The listing builds one solid part. Answer for the finished solid, in the listing's coordinates (mm). A direction names the side the tool comes from. Coordinates: 2 decimals unless noted, no trailing zeros. Order: outer loops, then holes, each group sorted by start corner. A loop starts at its lowest first (then second) coordinate and runs counter-clockwise, first axis right, second up. Notation, with made-up numbers: (25.5, -8.75) -> (45.5, -8.75) arc R13 cw to (45.5, 8.25) -> close; hole circle Ø3 at (54.5, -7). An arc over 180 degrees is marked (long way). Put each result on its own line as item: value. Start each with the question number.
```python
from build123d import *

# Parameters (mm, degrees)
BOSS_EXTRUDE1_DEPTH = 3.175
SKETCH2_R           = 1.6
CUT_EXTRUDE1_DEPTH  = 3.175


with BuildPart() as part:
    # Sketch1 → Boss-Extrude1 (new body)
    with BuildSketch(Plane.XY):
        Polygon((25, 7.5), (-25, 7.5), (-25, -7.5), (-17.5, -7.5), (-17.5, -10.675), (-12.5, -10.675), (-12.5, -7.5), (-2.5, -7.5), (-2.5, -10.675), (2.5, -10.675), (2.5, -7.5), (12.5, -7.5), (12.5, -10.675), (17.5, -10.675), (17.5, -7.5), (25, -7.5), align=None)
    extrude(amount=BOSS_EXTRUDE1_DEPTH)

    # Sketch2 → Cut-Extrude1 (cut)
    with BuildSketch(Plane.XY.offset(3.175)):
        with Locations((-18.4, 0)):
            Circle(SKETCH2_R)
        with Locations((18.4, 0)):
            Circle(SKETCH2_R)
    extrude(amount=-CUT_EXTRUDE1_DEPTH, mode=Mode.SUBTRACT)


solid = part.part
```
(1) Find the intervals of material crossed by L1, parallel to X at y = -9.25, z = 1.7; L2, parallel to Y at x = -18.4, z = 1.7; L3, parallel to X at y = 0.5, z = 2.95, in increasing order.
(2) The part is cut by section B-B on y = -9. Determine the outline of the cut face in (x, z) (3 decimals).
(3) Each of these flat-tipped pins is pushed along its axis until it touches: P1, Ø1, axis at y = -9.5, z = 2, coming from the +X side; P2, Ø1, axis at y = -9, z = 1.5, coming from the -X side; P3, Ø1, axis at x = 20, z = 2, coming from the -Y side. Where does it stop, or does it pass through?
(4) A tool of negligible diameter and unlimited length cuts with its end or side. For faces 1 (the flat face through (7, -7.5, 2)), 2 (the flat face through (-21, -7.5, 2)), 3 (the flat face through (0, 1, 0)), 4 (the flat face through (21, -7.5, 2)), from which of +Z, -Z, +X, -X, +Y, -Y can it reach the whole face along a straight path? Write none if from no direction.
(5) For a pull along X with two mould halves and no side action, classify faces 5 (the flat face through (17.5, -9, 2)), 6 (the flat face through (12.5, -9, 2)), 7 (the flat face through (-15, -10.675, 2)) as released by +X, released by -X, zero draft, split by the parting line, or undercut.
(6) The part is cut by section C-C on z = 2.6. Determine the outline of the cut face in (x, y) (3 decimals).
(7) The part is cut by section D-D on x = 19.5. Determine the outline of the cut face in (y, z) (3 decimals).
(8) The part is cut by section A-A on x = -18.4. Determine the outline of the cut face in (y, z) (3 decimals).
Worked out:
1. L1: -17.5 to -12.5, -2.5 to 2.5, 12.5 to 17.5
1. L2: -7.5 to -1.6, 1.6 to 7.5
1. L3: -25 to -19.92, -16.88 to 16.88, 19.92 to 25
2. outline: (-17.5, 0) -> (-12.5, 0) -> (-12.5, 3.175) -> (-17.5, 3.175) -> close; (-2.5, 0) -> (2.5, 0) -> (2.5, 3.175) -> (-2.5, 3.175) -> close; (12.5, 0) -> (17.5, 0) -> (17.5, 3.175) -> (12.5, 3.175) -> close
3. P1: x = 17.5
3. P2: x = -17.5
3. P3: y = -7.5
4. face 1: +Z, -Z, -Y
4. face 2: +Z, -Z, -X, -Y
4. face 3: -Z, +X, -X, +Y, -Y
4. face 4: +Z, -Z, +X, -Y
5. face 5: released by +X
5. face 6: undercut
5. face 7: zero draft
6. outline: (-25, -7.5) -> (-17.5, -7.5) -> (-17.5, -10.675) -> (-12.5, -10.675) -> (-12.5, -7.5) -> (-2.5, -7.5) -> (-2.5, -10.675) -> (2.5, -10.675) -> (2.5, -7.5) -> (12.5, -7.5) -> (12.5, -10.675) -> (17.5, -10.675) -> (17.5, -7.5) -> (25, -7.5) -> (25, 7.5) -> (-25, 7.5) -> close; hole circle Ø3.2 at (-18.4, 0); hole circle Ø3.2 at (18.4, 0)
7. outline: (-7.5, 0) -> (-1.162, 0) -> (-1.162, 3.175) -> (-7.5, 3.175) -> close; (1.162, 0) -> (7.5, 0) -> (7.5, 3.175) -> (1.162, 3.175) -> close
8. outline: (-7.5, 0) -> (-1.6, 0) -> (-1.6, 3.175) -> (-7.5, 3.175) -> close; (1.6, 0) -> (7.5, 0) -> (7.5, 3.175) -> (1.6, 3.175) -> close
